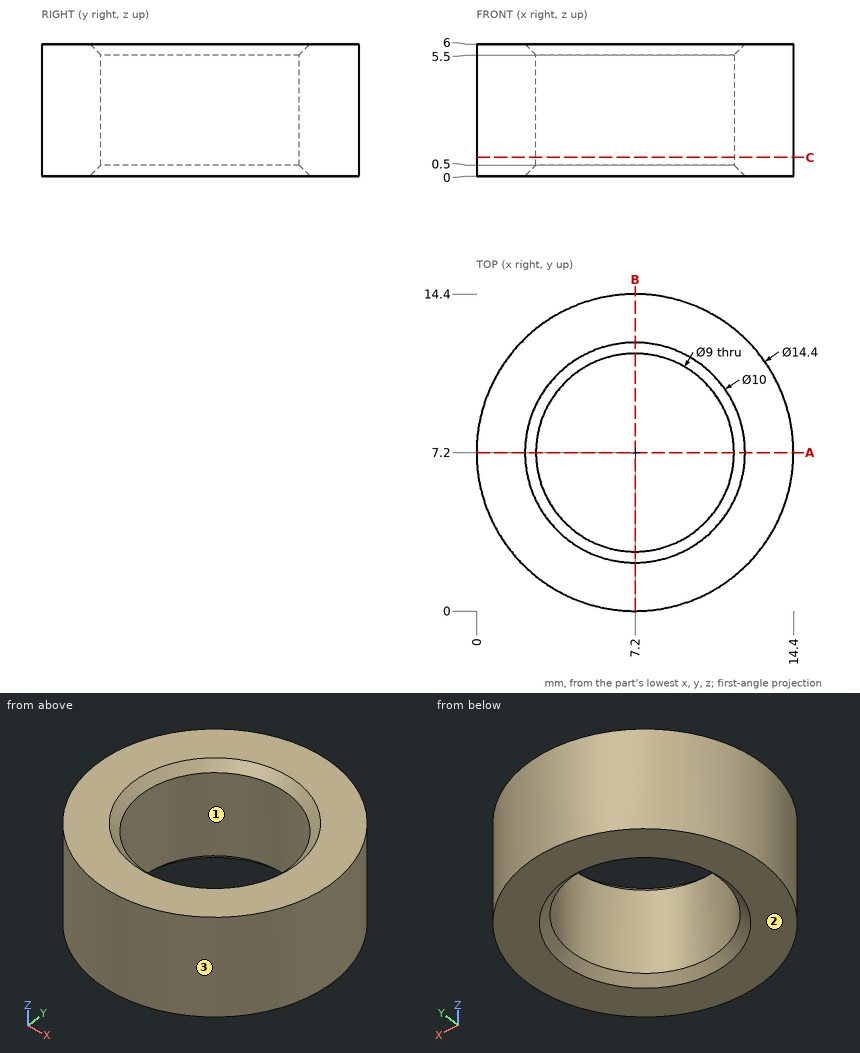
Geometry check sheet. Reference: drawing and pictorial views, mm from the part's lowest x, y, z. Coordinates: 2 decimals unless noted, no trailing zeros. Order: outer loops, then holes, each group sorted by start corner. A loop starts at its lowest first (then second) coordinate and runs counter-clockwise, first axis right, second up. Notation, with made-up numbers: (-21.5, -40) -> (1.5, -40) arc R20 ccw to (1.5, -3) -> close; hole circle Ø10 at (46.25, 74). An arc over 180 degrees is marked (long way). Put each result on its own line as item: value. Start each with the question number.
1) Release check for a two-part mould opening along Y. For the marked faces 1, 2 and 3 record: pulls with the +Y half, pulls with the -Y half, needs draft (parallel to the pull), parting line crosses it, or undercut.
2) Cross-section at C-C (z = 0.85). Enter the section's corners in (x, y).
3) Go/stop test with flat-tipped pins: pin 1 (3 mm diameter, centred on x = 7, z = 3, fed in from +Y); pin 2 (1.5 mm diameter, centred on y = 6, z = 1, fed in from -X). Record where each tip stops, or that it passes through.
4) Cross-section at A-A (y = 7.2). Enter the section's corners in (x, z), plus the area to 3 significant figures.
5) Material ranges on L1, parallel to Y at x = 7.2, z = 2.1; L2, parallel to Y at x = 3.25, z = 5.35; L3, parallel to X at y = 8, z = 1.95, recorded low to high.
Geometry check:
1. face 1: undercut
1. face 2: needs draft
1. face 3: parting line crosses it
2. outline: circle Ø14.4 at (7.2, 7.2); hole circle Ø9 at (7.2, 7.2)
3. pin 1: stops at y = 14.4
3. pin 2: stops at x = 0.01
4. outline: (0, 0) -> (2.2, 0) -> (2.7, 0.5) -> (2.7, 5.5) -> (2.2, 6) -> (0, 6) -> close; (11.7, 0.5) -> (12.2, 0) -> (14.4, 0) -> (14.4, 6) -> (12.2, 6) -> (11.7, 5.5) -> close
4. area: 31.9 mm^2
5. L1: y = 0 to 2.7, 11.7 to 14.4
5. L2: y = 1.18 to 5.04, 9.36 to 13.22
5. L3: x = 0.04 to 2.77, 11.63 to 14.36
